Part model, mm, in its own coordinate system. A direction names the side the tool comes from. Round coordinates to 2 decimals unless told otherwise and drop trailing zeros. Write each loop counter-clockwise with the first axis right and the second up, starting at its lowest first coordinate (ties: lowest second). Pieces come first, ordered by that corner, then holes.
```python
from build123d import *

# Parameters (mm, degrees)
BOSS_EXTRUDE1_DEPTH                                 = 50.8
SKETCH2_R                                           = 6.35
CUT_EXTRUDE1_DEPTH                                  = 51.8
LPATTERN1_COUNT                                     = 2
LPATTERN1_PITCH                                     = 76.2
LPATTERN1_COUNT_DIR2                                = 2
LPATTERN1_PITCH_DIR2                                = 63.5
CBORE_FOR_00_BINDING_HEAD_MACHINE_SCREW_D           = 5.08
CBORE_FOR_00_BINDING_HEAD_MACHINE_SCREW_CBORE_D     = 11.176
CBORE_FOR_00_BINDING_HEAD_MACHINE_SCREW_CBORE_DEPTH = 3.048
CUT_EXTRUDE6_DEPTH                                  = 5.08


with BuildPart() as part:
    # Sketch1 → Boss-Extrude1 (new body, symmetric)
    with BuildSketch(Plane.XY):
        with BuildLine():
            Line((25.4, 25.4), (50.8, 25.4))
            Line((50.8, 25.4), (50.8, -25.4))
            Line((50.8, -25.4), (-50.8, -25.4))
            Line((-50.8, -25.4), (-50.8, 25.4))
            Line((-50.8, 25.4), (-25.4, 25.4))
            ThreePointArc((-25.4, 25.4), (0, 0), (25.4, 25.4))
        make_face()
    extrude(amount=BOSS_EXTRUDE1_DEPTH, both=True)

    # Sketch2 → Cut-Extrude1 (cut, through all)
    with BuildSketch(Plane(origin=(0, 25.4, 0), x_dir=(1, 0, 0), z_dir=(0, 1, 0))):
        with Locations((-38.1, 31.75)):
            Circle(SKETCH2_R)
    cut_extrude1 = extrude(amount=-CUT_EXTRUDE1_DEPTH, mode=Mode.SUBTRACT)

    # LPattern1: Cut-Extrude1 2 × 2
    with Locations(*[(i * LPATTERN1_PITCH, 0, j * LPATTERN1_PITCH_DIR2) for i in range(LPATTERN1_COUNT) for j in range(LPATTERN1_COUNT_DIR2) if (i, j) != (0, 0)]):
        add(cut_extrude1, mode=Mode.SUBTRACT)

    # CBORE for #00 Binding Head Machine Screw1 (through all)
    with Locations(Plane.XY.offset(50.8)):
        with Locations((-25.4, -12.7), (25.4, -12.7)):
            CounterBoreHole(CBORE_FOR_00_BINDING_HEAD_MACHINE_SCREW_D / 2, CBORE_FOR_00_BINDING_HEAD_MACHINE_SCREW_CBORE_D / 2, CBORE_FOR_00_BINDING_HEAD_MACHINE_SCREW_CBORE_DEPTH)

    # Sketch7 → Cut-Extrude6 (cut)
    with BuildSketch(Plane(origin=(50.8, 0, 0), x_dir=(0, 0, -1), z_dir=(1, 0, 0))):
        with BuildLine():
            Line((-25.4, 6.35), (25.4, 6.35))
            ThreePointArc((25.4, 6.35), (31.75, 0), (25.4, -6.35))
            Line((25.4, -6.35), (-25.4, -6.35))
            ThreePointArc((-25.4, -6.35), (-31.75, 0), (-25.4, 6.35))
        make_face()
    extrude(amount=-CUT_EXTRUDE6_DEPTH, mode=Mode.SUBTRACT)


solid = part.part
```
Q1. Drop flat-ended pins along their axis: pin 1 (6.5 mm diameter, centred on x = 25.4, y = -12.7, fed in from +Z); pin 2 (7.5 mm diameter, centred on x = -38.1, z = -31.75, fed in from +Y); pin 3 (4 mm diameter, centred on x = -4, z = -0.5, fed in from +Y); pin 4 (1.5 mm diameter, centred on y = -5, z = 12, fed in from +X). Give the stop position or say it passes through.
Values follow:
pin 1: stops at z = 47.75
pin 2: passes through
pin 3: stops at y = 0.72
pin 4: stops at x = 45.72
Q2. Mould opens along X. For faces 4 (the cylindrical face through (27.938, -12.588, -2.214)), 5 (the cylindrical face through (-32.043, 0.356, 29.843)), 6 (the flat face through (45.72, 0, 0)), 7 (the flat face through (1, -25.4, 1)) say: +X half, -X half, draft (parallel to the pull), parting line (faces both ways), or undercut.
Values follow:
face 4: undercut
face 5: undercut
face 6: +X half
face 7: draft
Q3. Wall check: L1, parallel to Z at x = 38.1, y = -3; L2, parallel to X at y = -12.5, z = 31.75; L3, parallel to X at y = -7, z = 31.75. Give the ranges that are in metal, low to high.
Values follow:
L1: z = -50.8 to -38.1, -25.4 to 25.4, 38.1 to 50.8
L2: x = -50.8 to -44.45, -31.75 to -27.93, -22.87 to 22.87, 27.93 to 31.75, 44.45 to 50.8
L3: x = -50.8 to -44.45, -31.75 to 31.75, 44.45 to 50.8
Q4. Which spindle directions (+Z, -Z, +X, -X, +Y, -Y) get a long thin tool onto all of the face, cutting with end or side? Do faces 1 (the flat face through (28, -14, 47.752)), 2 (the flat face through (-50.8, 0, 1)), 3 (the flat face through (48, -6.35, 0)). Say none if no direction does.
Values follow:
face 1: +Z
face 2: +Z, -Z, -X, +Y, -Y
face 3: +X
Q5. Cut at D-D on y = 4. Write the cut outline in (x, z), plus the area to 3 significant figures.
Values follow:
outline: (-50.8, -50.8) - (-13.68, -50.8) - (-13.68, 50.8) - (-50.8, 50.8) - close; (13.68, -50.8) - (50.8, -50.8) - (50.8, -30.33) - (45.72, -30.33) - (45.72, 30.33) - (50.8, 30.33) - (50.8, 50.8) - (13.68, 50.8) - close; hole circle Ø12.7 at (-38.1, -31.75); hole circle Ø12.7 at (-38.1, 31.75); hole circle Ø12.7 at (38.1, -31.75); hole circle Ø12.7 at (38.1, 31.75)
area: 6,730 mm2
Q6. Cut at A-A on y = -12.7. Write the cut outline in (x, z).
Values follow:
outline: (-50.8, -50.8) - (-27.94, -50.8) - (-27.94, 47.75) - (-30.99, 47.75) - (-30.99, 50.8) - (-50.8, 50.8) - close; (-22.86, -50.8) - (22.86, -50.8) - (22.86, 47.75) - (19.81, 47.75) - (19.81, 50.8) - (-19.81, 50.8) - (-19.81, 47.75) - (-22.86, 47.75) - close; (27.94, -50.8) - (50.8, -50.8) - (50.8, 50.8) - (30.99, 50.8) - (30.99, 47.75) - (27.94, 47.75) - close; hole circle Ø12.7 at (-38.1, -31.75); hole circle Ø12.7 at (-38.1, 31.75); hole circle Ø12.7 at (38.1, -31.75); hole circle Ø12.7 at (38.1, 31.75)
Q7. Cut at B-B on z = -24. Write the cut outline in (x, y).
Values follow:
outline: (-50.8, -25.4) - (50.8, -25.4) - (50.8, -6.35) - (45.72, -6.35) - (45.72, 6.35) - (50.8, 6.35) - (50.8, 25.4) - (25.4, 25.4) arc R25.4 cw to (-25.4, 25.4) - (-50.8, 25.4) - close; hole circle Ø5.08 at (-25.4, -12.7); hole circle Ø5.08 at (25.4, -12.7)
Q8. Cut at C-C on x = -38.1. Write the cut outline in (y, z).
Values follow:
outline: (-25.4, -50.8) - (25.4, -50.8) - (25.4, -38.1) - (-25.4, -38.1) - close; (-25.4, -25.4) - (25.4, -25.4) - (25.4, 25.4) - (-25.4, 25.4) - close; (-25.4, 38.1) - (25.4, 38.1) - (25.4, 50.8) - (-25.4, 50.8) - close
